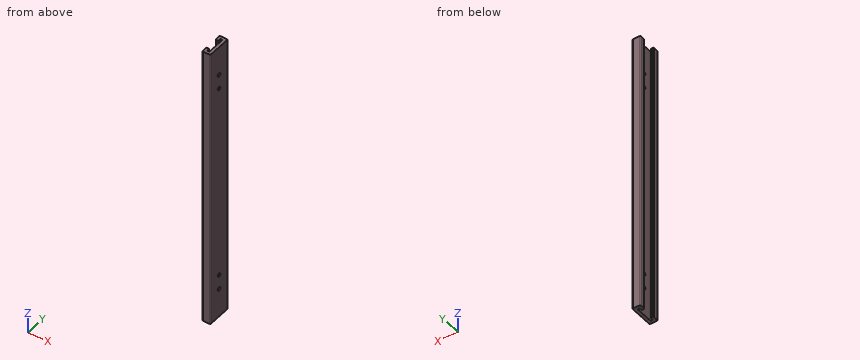
```python
from build123d import *

# Parameters (mm, degrees)
BOSS_EXTRUDE1_DEPTH = 195
CUT_EXTRUDE1_REACH  = 197.813
SKETCH2_R           = 2.5


with BuildPart() as part:
    # Sketch1 → Boss-Extrude1 (new, symmetric)
    with BuildSketch(Plane.XY):
        with BuildLine():
            Line((5.5, -15.5), (5.5, 15.5))
            ThreePointArc((5.5, 15.5), (5.207106781, 16.207106781), (4.5, 16.5))
            Line((4.5, 16.5), (-4.5, 16.5))
            ThreePointArc((-4.5, 16.5), (-5.207106781, 16.207106781), (-5.5, 15.5))
            Line((-5.5, 15.5), (-5.5, 9.5))
            ThreePointArc((-5.5, 9.5), (-5.207106781, 8.792893219), (-4.5, 8.5))
            Line((-4.5, 8.5), (-2.75, 8.5))
            ThreePointArc((-2.75, 8.5), (-2.042893219, 8.792893219), (-1.75, 9.5))
            Line((-1.75, 9.5), (-1.75, 11.5))
            ThreePointArc((-1.75, 11.5), (-1.457106781, 12.207106781), (-0.75, 12.5))
            Line((-0.75, 12.5), (0.25, 12.5))
            ThreePointArc((0.25, 12.5), (0.957106781, 12.207106781), (1.25, 11.5))
            Line((1.25, 11.5), (1.25, -11.5))
            ThreePointArc((1.25, -11.5), (0.957106781, -12.207106781), (0.25, -12.5))
            Line((0.25, -12.5), (-0.75, -12.5))
            ThreePointArc((-0.75, -12.5), (-1.457106781, -12.207106781), (-1.75, -11.5))
            Line((-1.75, -11.5), (-1.75, -9.5))
            ThreePointArc((-1.75, -9.5), (-2.042893219, -8.792893219), (-2.75, -8.5))
            Line((-2.75, -8.5), (-4.5, -8.5))
            ThreePointArc((-4.5, -8.5), (-5.207106781, -8.792893219), (-5.5, -9.5))
            Line((-5.5, -9.5), (-5.5, -15.5))
            ThreePointArc((-5.5, -15.5), (-5.207106781, -16.207106781), (-4.5, -16.5))
            Line((-4.5, -16.5), (4.5, -16.5))
            ThreePointArc((4.5, -16.5), (5.207106781, -16.207106781), (5.5, -15.5))
        make_face()
    extrude(amount=BOSS_EXTRUDE1_DEPTH, both=True)

    # Sketch2 → Cut-Extrude1 (cut, up to next)
    with BuildSketch(Plane.ZY.offset(-1.25), mode=Mode.PRIVATE) as cut_extrude1_sk1:
        with Locations((155, 0)):
            Circle(SKETCH2_R)
    cut_extrude1_tool1 = extrude(cut_extrude1_sk1.sketch, amount=-CUT_EXTRUDE1_REACH, mode=Mode.PRIVATE) & part.part
    # Sketch2 → Cut-Extrude1 (cut, up to next)
    with BuildSketch(Plane.ZY.offset(-1.25), mode=Mode.PRIVATE) as cut_extrude1_sk2:
        with Locations((135, 0)):
            Circle(SKETCH2_R)
    cut_extrude1_tool2 = extrude(cut_extrude1_sk2.sketch, amount=-CUT_EXTRUDE1_REACH, mode=Mode.PRIVATE) & part.part
    # Sketch2 → Cut-Extrude1 (cut, up to next)
    with BuildSketch(Plane.ZY.offset(-1.25), mode=Mode.PRIVATE) as cut_extrude1_sk3:
        with Locations((-135, 0)):
            Circle(SKETCH2_R)
    cut_extrude1_tool3 = extrude(cut_extrude1_sk3.sketch, amount=-CUT_EXTRUDE1_REACH, mode=Mode.PRIVATE) & part.part
    # Sketch2 → Cut-Extrude1 (cut, up to next)
    with BuildSketch(Plane.ZY.offset(-1.25), mode=Mode.PRIVATE) as cut_extrude1_sk4:
        with Locations((-155, 0)):
            Circle(SKETCH2_R)
    cut_extrude1_tool4 = extrude(cut_extrude1_sk4.sketch, amount=-CUT_EXTRUDE1_REACH, mode=Mode.PRIVATE) & part.part
    add(cut_extrude1_tool1.solids().sort_by_distance((1.25, 0, 155))[0], mode=Mode.SUBTRACT)
    add(cut_extrude1_tool2.solids().sort_by_distance((1.25, 0, 135))[0], mode=Mode.SUBTRACT)
    add(cut_extrude1_tool3.solids().sort_by_distance((1.25, 0, -135))[0], mode=Mode.SUBTRACT)
    add(cut_extrude1_tool4.solids().sort_by_distance((1.25, 0, -155))[0], mode=Mode.SUBTRACT)


solid = part.part
```
The listing builds one solid part. Answer for the finished solid, in the listing's coordinates (mm). Give positions to 0.01 mm unless a question says otherwise; leave off trailing zeros. Order: outer loops, then holes, each group sorted by start corner. A loop starts at its lowest first (then second) coordinate and runs counter-clockwise, first axis right, second up. Notation, with made-up numbers: (-17.75, 64.5) - (28.25, 64.5) arc R22 ccw to (28.25, 71.5) - close; hole circle Ø10 at (-24.75, 60). An arc over 180 degrees is marked (long way). Use one line per item in the form item = value. Start each with the question number.
(1) Consider line 1 (Y direction, x = -3.75, z = -123); line 2 (X direction, y = 10, z = -126.5); line 3 (Y direction, x = 3.15, z = 155). Determine where each line is inside the solid, lowest interval first. Write a range as from..to.
(2) A cutting plane is placed at A-A, the plane z = 81. Write down the section's boundary in (x, y).
(3) Flat-ended cylindrical pins translate along their axes: pin 1 Ø6 at (y, z) = (3.5, 83.5) entering from -X; pin 2 Ø3 at (y, z) = (0, -135) entering from +X. Find the tip coordinate at first contact, or state that the pin passes through.
Ans:
q1.line_1 = -16.5..-8.5, 8.5..16.5
q1.line_2 = -5.5..-1.75, 1.25..5.5
q1.line_3 = -16.5..-2.5, 2.5..16.5
q2.outline = (-5.5, -15.5) arc R1 ccw to (-4.5, -16.5) - (4.5, -16.5) arc R1 ccw to (5.5, -15.5) - (5.5, 15.5) arc R1 ccw to (4.5, 16.5) - (-4.5, 16.5) arc R1 ccw to (-5.5, 15.5) - (-5.5, 9.5) arc R1 ccw to (-4.5, 8.5) - (-2.75, 8.5) arc R1 ccw to (-1.75, 9.5) - (-1.75, 11.5) arc R1 cw to (-0.75, 12.5) - (0.25, 12.5) arc R1 cw to (1.25, 11.5) - (1.25, -11.5) arc R1 cw to (0.25, -12.5) - (-0.75, -12.5) arc R1 cw to (-1.75, -11.5) - (-1.75, -9.5) arc R1 ccw to (-2.75, -8.5) - (-4.5, -8.5) arc R1 ccw to (-5.5, -9.5) - close
q3.pin_1 = 1.25
q3.pin_2 = through
